Design review of the part built by this model. Coordinates are the model's own, in mm. A direction names the side the tool comes from. Coordinates: 2 decimals unless noted, no trailing zeros. Write each loop counter-clockwise with the first axis right and the second up, starting at its lowest first coordinate (ties: lowest second). Pieces come first, ordered by that corner, then holes. Notation, with made-up numbers: (26, 71.5) -> (58, 71.5) arc R17 cw to (58, 97.5) -> close; hole circle Ø4 at (51.5, 85.25). An arc over 180 degrees is marked (long way). Write item = value, one per line. Start each with the question number.
```python
from build123d import *

# Parameters (mm, degrees)
SKETCH_W     = 10
SKETCH_H     = 51
SKETCH_R     = 2.25
PAD_DEPTH    = 3
FILLET_R     = 4
SKETCH001_W  = 15
SKETCH001_H  = 3
PAD001_DEPTH = 2.5
SKETCH002_W  = 15
SKETCH002_H  = 3
PAD002_DEPTH = 2.5
FILLET001_R  = 2


with BuildPart() as part:
    # Sketch → Pad (new body)
    with BuildSketch(Plane.XY):
        with Locations((5, 25.5)):
            Rectangle(SKETCH_W, SKETCH_H)
        with Locations((5, 45)):
            Circle(SKETCH_R, mode=Mode.SUBTRACT)
        with Locations((5, 10)):
            Circle(SKETCH_R, mode=Mode.SUBTRACT)
    extrude(amount=PAD_DEPTH)

    # Fillet
    fillet_edges = [part.edges().sort_by_distance(p)[0] for p in [
        (0, 51, 1.5),
        (10, 51, 1.5),
    ]]
    fillet(fillet_edges, radius=FILLET_R)

    # Sketch001 (on Face7 of Fillet) → Pad001 (join)
    with BuildSketch(Plane(origin=(0, 0, 0), x_dir=(0, -1, 0), z_dir=(-1, 0, 0))):
        with Locations((-7.5, 1.5)):
            Rectangle(SKETCH001_W, SKETCH001_H)
    extrude(amount=PAD001_DEPTH)

    # Sketch002 (on Face1 of Pad001) → Pad002 (join)
    with BuildSketch(Plane.YZ.offset(10)):
        with Locations((7.5, 1.5)):
            Rectangle(SKETCH002_W, SKETCH002_H)
    extrude(amount=PAD002_DEPTH)

    # Fillet001
    fillet001_edges = [part.edges().sort_by_distance(p)[0] for p in [
        (0, 15, 1.5),
        (10, 15, 1.5),
    ]]
    fillet(fillet001_edges, radius=FILLET001_R)


solid = part.part
```
(1) Take a section at A-A, the plane y = 45. State the section outline as (x, z) points.
(2) For line 1 (Y direction, x = 5, z = 1.8); line 2 (Y direction, x = 4, z = 1.05); line 3 (X direction, y = 19, z = 2.85), list the stretches that pass through material, from the lowest coordinate up.
(3) For faces 1 (the face through (10, 32, 1)), 2 (the face through (0, 32, 1)), 3 (the face through (5, 25, 0)), list the 3-axis set-ups (+Z, -Z, +X, -X, +Y, -Y) from which the entire face can be reached by the end or side of a thin tool; tool diameter is ignored.
(4) For pin 1 Ø2 at (x, y) = (6.5, 27.5) entering from -Z; pin 2 Ø1.5 at (y, z) = (29.5, 1) entering from +X; pin 3 Ø1.5 at (y, z) = (30.5, 1) entering from -X; pin 4 Ø3.5 at (x, y) = (5, 45) entering from -Z, all flat-tipped, find the tip position at first contact; note any pin that passes through.
(5) Mouldability with a two-part tool opening along X and no side actions: class faces 4 (the face through (5, 0, 1)), 5 (the face through (1.141, 49.797, 1.521)), 6 (the face through (4.71, 47.23, 1.48)) as pulls with the +X half, pulls with the -X half, needs draft (parallel to the pull), parting line crosses it, or undercut.
(6) Take a section at B-B, the plane z = 1.8. State the section outline as (x, y) points, then the cut area to 3 significant figures.
(7) Take a section at C-C, the plane x = 5. State the section outline as (y, z) points.
(8) Take a section at D-D, the plane y = 10. State the section outline as (x, z) points.
Report:
q1.outline = (0, 0) -> (2.75, 0) -> (2.75, 3) -> (0, 3) -> close; (7.25, 0) -> (10, 0) -> (10, 3) -> (7.25, 3) -> close
q2.line_1 = 0 to 7.75, 12.25 to 42.75, 47.25 to 51
q2.line_2 = 0 to 7.98, 12.02 to 42.98, 47.02 to 51
q2.line_3 = 0 to 10
q3.face_1 = +Z, -Z, +X, +Y
q3.face_2 = +Z, -Z, -X, +Y
q3.face_3 = -Z, +X, -X, +Y, -Y
q4.pin_1 = 0
q4.pin_2 = 10
q4.pin_3 = 0
q4.pin_4 = through
q5.face_4 = needs draft
q5.face_5 = pulls with the -X half
q5.face_6 = undercut
q6.outline = (-2.5, 0) -> (12.5, 0) -> (12.5, 15) -> (12, 15) arc R2 cw to (10, 17) -> (10, 47) arc R4 ccw to (6, 51) -> (4, 51) arc R4 ccw to (0, 47) -> (0, 17) arc R2 cw to (-2, 15) -> (-2.5, 15) -> close; hole circle Ø4.5 at (5, 10); hole circle Ø4.5 at (5, 45)
q6.area = 548 mm2
q7.outline = (0, 0) -> (7.75, 0) -> (7.75, 3) -> (0, 3) -> close; (12.25, 0) -> (42.75, 0) -> (42.75, 3) -> (12.25, 3) -> close; (47.25, 0) -> (51, 0) -> (51, 3) -> (47.25, 3) -> close
q8.outline = (-2.5, 0) -> (2.75, 0) -> (2.75, 3) -> (-2.5, 3) -> close; (7.25, 0) -> (12.5, 0) -> (12.5, 3) -> (7.25, 3) -> close
